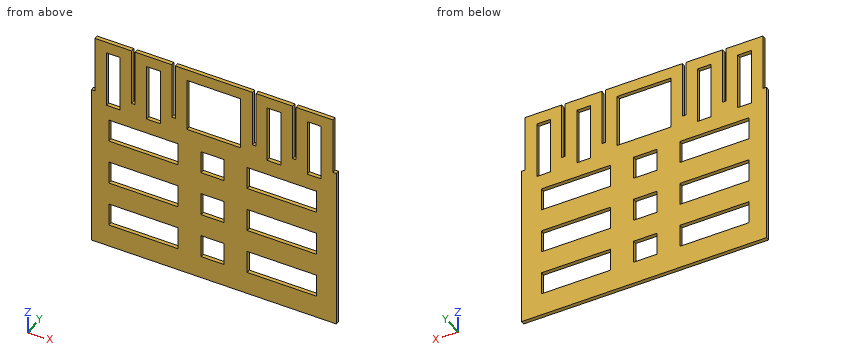
Autodesk Inventor part; units mm, degrees
ref_plane "YZ Plane" through (0, 0, 0) normal (1, 0, 0) x (0, 1, 0)
ref_plane "XZ Plane" through (0, 0, 0) normal (0, 1, 0) x (-1, 0, 0)
ref_plane "XY Plane" through (0, 0, 0) normal (0, 0, 1) x (1, 0, 0)
sketch "Sketch1" plane through (0, 0, 0) normal (0, 1, 0) x (-1, 0, 0)
  line L0 (0, 0) -> (318.5, 0)
  line L1 (318.5, 0) -> (318.5, -290)
  line L2 (318.5, -290) -> (0, -290)
  line L3 (0, -290) -> (0, 0)
  dimension "d0" = 318.5
  dimension "d1" = 290
extrude "Extrusion1" add sketch "Sketch1" along normal blind 5
sketch "Sketch2" plane through (0, 5, 0) normal (0, 1, 0) x (1, 0, 0)
  line L0 (0, 290) -> (-318.5, 290)
  line L1 (-318.5, 290) -> (-318.5, 75)
  line L2 (-318.5, 290) -> (-318.5, 0)
  line L3 (-318.5, 0) -> (0, 0)
  line L4 (-318.5, 75) -> (-314, 75)
  line L5 (-314, 75) -> (-314, 0)
  line L6 (-314, 0) -> (-318.5, 0)
  line L7 (-318.5, 0) -> (-318.5, 75)
  line L8 (-314, 75) -> (-266.25, 75)
  line L9 (-266.25, 75) -> (-261.75, 75)
  line L10 (-261.75, 75) -> (-261.75, 0)
  line L11 (-261.75, 0) -> (-266.25, 0)
  line L12 (-266.25, 0) -> (-266.25, 75)
  line L13 (-261.75, 75) -> (-214, 75)
  line L14 (-214, 75) -> (-209.5, 75)
  line L15 (-209.5, 75) -> (-209.5, 0)
  line L16 (-209.5, 0) -> (-214, 0)
  line L17 (-214, 0) -> (-214, 75)
  line L18 (-209.5, 75) -> (-162.03, 75)
  line L19 (-159.25, 290) -> (-159.25, 0)
  line L20 (0, 75) -> (-4.5, 75)
  line L21 (-4.5, 75) -> (-4.5, 0)
  line L22 (-4.5, 0) -> (0, 0)
  line L23 (0, 0) -> (0, 75)
  line L24 (-4.5, 75) -> (-52.25, 75)
  line L25 (-52.25, 75) -> (-56.75, 75)
  line L26 (-56.75, 75) -> (-56.75, 0)
  line L27 (-56.75, 0) -> (-52.25, 0)
  line L28 (-52.25, 0) -> (-52.25, 75)
  line L29 (-56.75, 75) -> (-104.5, 75)
  line L30 (-104.5, 75) -> (-109, 75)
  line L31 (-109, 75) -> (-109, 0)
  line L32 (-109, 0) -> (-104.5, 0)
  line L33 (-104.5, 0) -> (-104.5, 75)
  point P0 (-214, 0)
  point P1 (-266.25, 0)
  dimension "d4" = 215
  dimension "d5" = 4.5
  dimension "d6" = 47.75
  dimension "d7" = 4.5
  dimension "d8" = 47.75
  dimension "d9" = 4.5
  dimension "d10" = 47.47
extrude "Extrusion2" cut sketch "Sketch2" against normal blind 5 contours L31 L30 L33 L3 | L4 L5 L3 L2 | L3 L17 L14 L15 | L9 L10 L3 L12 | L26 L25 L28 L3 | L21 L20 L23 L3
sketch "Sketch3" plane through (0, 5, 0) normal (0, 1, 0) x (1, 0, 0)
  line L0 (-318.5, 290) -> (-318.5, 75)
  line L1 (-318.5, 290) -> (-296, 290)
  line L2 (-296, 290) -> (-296, 260)
  line L3 (-296, 260) -> (-318.5, 260)
  line L4 (-318.5, 260) -> (-318.5, 290)
  line L5 (-296, 260) -> (-266, 260)
  line L6 (-266, 260) -> (-266, 230)
  line L7 (-266, 230) -> (-296, 230)
  line L8 (-296, 230) -> (-296, 260)
  line L9 (-266, 200) -> (-266, 170)
  line L10 (-266, 170) -> (-296, 170)
  line L11 (-296, 170) -> (-296, 200)
  line L12 (-296, 200) -> (-266, 200)
  line L13 (-266, 140) -> (-266, 110)
  line L14 (-266, 110) -> (-296, 110)
  line L15 (-296, 110) -> (-296, 140)
  line L16 (-296, 140) -> (-266, 140)
  line L17 (-206, 260) -> (-206, 230)
  line L18 (-206, 230) -> (-236, 230)
  line L19 (-236, 230) -> (-236, 260)
  line L20 (-236, 260) -> (-206, 260)
  line L21 (-206, 200) -> (-206, 170)
  line L22 (-206, 170) -> (-236, 170)
  line L23 (-236, 170) -> (-236, 200)
  line L24 (-236, 200) -> (-206, 200)
  line L25 (-206, 140) -> (-206, 110)
  line L26 (-206, 110) -> (-236, 110)
  line L27 (-236, 110) -> (-236, 140)
  line L28 (-236, 140) -> (-206, 140)
  line L29 (-146, 260) -> (-146, 230)
  line L30 (-146, 230) -> (-176, 230)
  line L31 (-176, 230) -> (-176, 260)
  line L32 (-176, 260) -> (-146, 260)
  line L33 (-146, 200) -> (-146, 170)
  line L34 (-146, 170) -> (-176, 170)
  line L35 (-176, 170) -> (-176, 200)
  line L36 (-176, 200) -> (-146, 200)
  line L37 (-146, 140) -> (-146, 110)
  line L38 (-146, 110) -> (-176, 110)
  line L39 (-176, 110) -> (-176, 140)
  line L40 (-176, 140) -> (-146, 140)
  line L41 (-86, 260) -> (-86, 230)
  line L42 (-86, 230) -> (-116, 230)
  line L43 (-116, 230) -> (-116, 260)
  line L44 (-116, 260) -> (-86, 260)
  line L45 (-86, 200) -> (-86, 170)
  line L46 (-86, 170) -> (-116, 170)
  line L47 (-116, 170) -> (-116, 200)
  line L48 (-116, 200) -> (-86, 200)
  line L49 (-86, 140) -> (-86, 110)
  line L50 (-86, 110) -> (-116, 110)
  line L51 (-116, 110) -> (-116, 140)
  line L52 (-116, 140) -> (-86, 140)
  line L53 (-26, 260) -> (-26, 230)
  line L54 (-26, 230) -> (-56, 230)
  line L55 (-56, 230) -> (-56, 260)
  line L56 (-56, 260) -> (-26, 260)
  line L57 (-26, 200) -> (-26, 170)
  line L58 (-26, 170) -> (-56, 170)
  line L59 (-56, 170) -> (-56, 200)
  line L60 (-56, 200) -> (-26, 200)
  line L61 (-26, 140) -> (-26, 110)
  line L62 (-26, 110) -> (-56, 110)
  line L63 (-56, 110) -> (-56, 140)
  line L64 (-56, 140) -> (-26, 140)
  line L65 (-266, 200) -> (-236, 200)
  line L66 (-236, 200) -> (-236, 170)
  line L67 (-236, 170) -> (-266, 170)
  line L68 (-266, 170) -> (-266, 200)
  line L69 (-86, 200) -> (-56, 200)
  line L70 (-56, 200) -> (-56, 170)
  line L71 (-56, 170) -> (-86, 170)
  line L72 (-86, 170) -> (-86, 200)
  line L73 (-86, 260) -> (-56, 260)
  line L74 (-56, 260) -> (-56, 230)
  line L75 (-56, 230) -> (-86, 230)
  line L76 (-86, 230) -> (-86, 260)
  line L77 (-266, 260) -> (-236, 260)
  line L78 (-236, 260) -> (-236, 230)
  line L79 (-236, 230) -> (-266, 230)
  line L80 (-266, 230) -> (-266, 260)
  line L81 (-266, 140) -> (-236, 140)
  line L82 (-236, 140) -> (-236, 110)
  line L83 (-236, 110) -> (-266, 110)
  line L84 (-266, 110) -> (-266, 140)
  line L85 (-86, 140) -> (-56, 140)
  line L86 (-56, 140) -> (-56, 110)
  line L87 (-56, 110) -> (-86, 110)
  line L88 (-86, 110) -> (-86, 140)
  line L89 (-209.5, 0) -> (-109, 0)
  line L90 (-209.5, 0) -> (-194.5, 0)
  line L91 (-194.5, 0) -> (-194.5, 15)
  line L92 (-194.5, 15) -> (-209.5, 15)
  line L93 (-209.5, 15) -> (-209.5, 0)
  line L94 (-194.5, 15) -> (-124.5, 15)
  line L95 (-124.5, 15) -> (-124.5, 85)
  line L96 (-124.5, 85) -> (-194.5, 85)
  line L97 (-194.5, 85) -> (-194.5, 15)
  line L98 (-314, 0) -> (-314, 75)
  line L99 (-314, 0) -> (-299, 0)
  line L100 (-299, 0) -> (-299, 15)
  line L101 (-299, 15) -> (-314, 15)
  line L102 (-314, 15) -> (-314, 0)
  line L103 (-266.25, 75) -> (-266.25, 0)
  line L104 (-266.25, 75) -> (-281.25, 75)
  line L105 (-281.25, 75) -> (-281.25, 90)
  line L106 (-281.25, 90) -> (-266.25, 90)
  line L107 (-266.25, 90) -> (-266.25, 75)
  line L108 (-281.25, 90) -> (-299, 90)
  line L109 (-299, 90) -> (-299, 15)
  line L110 (-299, 15) -> (-281.25, 15)
  line L111 (-281.25, 15) -> (-281.25, 90)
  line L112 (-229, 15) -> (-229, 90)
  line L113 (-246.75, 90) -> (-246.75, 15)
  line L114 (-246.75, 15) -> (-229, 15)
  line L115 (-229, 90) -> (-246.75, 90)
  line L116 (-176.75, 15) -> (-176.75, 90)
  line L117 (-194.5, 90) -> (-194.5, 15)
  line L118 (-194.5, 15) -> (-176.75, 15)
  line L119 (-176.75, 90) -> (-194.5, 90)
  line L120 (-124.5, 15) -> (-124.5, 90)
  line L121 (-142.25, 90) -> (-142.25, 15)
  line L122 (-142.25, 15) -> (-124.5, 15)
  line L123 (-124.5, 90) -> (-142.25, 90)
  line L124 (-72.25, 15) -> (-72.25, 90)
  line L125 (-90, 90) -> (-90, 15)
  line L126 (-90, 15) -> (-72.25, 15)
  line L127 (-72.25, 90) -> (-90, 90)
  line L128 (-20, 15) -> (-20, 90)
  line L129 (-37.75, 90) -> (-37.75, 15)
  line L130 (-37.75, 15) -> (-20, 15)
  line L131 (-20, 90) -> (-37.75, 90)
  point P0 (-209.5, 75)
  dimension "d25" = 22.5
  dimension "d26" = 30
  dimension "d27" = 30
  dimension "d28" = 30
  dimension "d31" = 60
  dimension "d34" = 60
  dimension "d37" = 15
  dimension "d38" = 15
  dimension "d39" = 70
  dimension "d40" = 70
  dimension "d41" = 15
  dimension "d42" = 15
  dimension "d43" = 15
  dimension "d44" = 15
  dimension "d47" = 52.25
extrude "Extrusion3" cut sketch "Sketch3" against normal blind 5 contours L5 L6 L7 L8 | L77 L19 L79 L6 | L20 L17 L18 L19 | L65 L23 L67 L9 | L9 L10 L11 L12 | L24 L21 L22 L23 | L81 L27 L83 L13 | L13 L14 L15 L16 | L28 L25 L26 L27 | L29 L30 L31 L32 | L33 L34 L35 L36 | L37 L38 L39 L40 | L73 L55 L75 L41 | L41 L42 L43 L44 | L56 L53 L54 L55 | L69 L59 L71 L45 | L45 L46 L47 L48 | L60 L57 L58 L59 | L85 L63 L87 L49 | L49 L50 L51 L52 | L64 L61 L62 L63 | L97 L96 L116 L94 | L116 L96 L121 L94 | L121 L96 L95 L94 | L109 L108 L105 L111 L110 | L114 L113 L115 L112 | L126 L125 L127 L124 | L130 L129 L131 L128
properties part number "backrest" material "Foam Core Board"
Part model, mm, in its own coordinate system. Coordinates: 2 decimals unless noted, no trailing zeros. Write each loop counter-clockwise with the first axis right and the second up, starting at its lowest first coordinate (ties: lowest second). Pieces come first, ordered by that corner, then holes. Notation, with made-up numbers: (83.25, 64.5) - (125.25, 64.5) arc R15 ccw to (125.25, 68.5) - close; hole circle Ø5 at (89.25, 66). An arc over 180 degrees is marked (long way). Put each result on its own line as item: value.
1. Band-saw the part on A-A (x = -276.5). Write the cut outline in (y, z), then the cut area to 3 significant figures.
Final values:
outline: (0, -290) - (5, -290) - (5, -260) - (0, -260) - close; (0, -230) - (5, -230) - (5, -200) - (0, -200) - close; (0, -170) - (5, -170) - (5, -140) - (0, -140) - close; (0, -110) - (5, -110) - (5, 0) - (0, 0) - close
area: 1,000 mm²
2. Probe line 1 along Z through (x, y) = (-258.5, 3.65); line 2 along Z through (x, y) = (-293.5, 3.3); line 3 along X through (y, z) = (0.7, -190.5). List the from-to ranges inside material, lowest first. Write a range as [from, to].
Final values:
line 1: z = [-290, -260], [-230, -200], [-170, -140], [-110, 0]
line 2: z = [-290, -260], [-230, -200], [-170, -140], [-110, -90], [-15, 0]
line 3: x = [-318.5, -296], [-206, -176], [-146, -116], [-26, 0]
3. Band-saw the part on B-B (z = -78.5). Write the cut outline in (x, y).
Final values:
outline: (-318.5, 0) - (-299, 0) - (-299, 5) - (-318.5, 5) - close; (-281.25, 0) - (-246.75, 0) - (-246.75, 5) - (-281.25, 5) - close; (-229, 0) - (-194.5, 0) - (-194.5, 5) - (-229, 5) - close; (-124.5, 0) - (-90, 0) - (-90, 5) - (-124.5, 5) - close; (-72.25, 0) - (-37.75, 0) - (-37.75, 5) - (-72.25, 5) - close; (-20, 0) - (0, 0) - (0, 5) - (-20, 5) - close
4. Flat gauge pin, fed straight in: pin 1 Ø1.5 at (y, z) = (0.5, -49) entering from +X. Where does the tip first touch, or does it go through?
Final values:
pin 1: stops at x = -4.5
5. Band-saw the part on C-C (z = -128.5). Write the cut outline in (x, y).
Final values:
outline: (-318.5, 0) - (-296, 0) - (-296, 5) - (-318.5, 5) - close; (-206, 0) - (-176, 0) - (-176, 5) - (-206, 5) - close; (-146, 0) - (-116, 0) - (-116, 5) - (-146, 5) - close; (-26, 0) - (0, 0) - (0, 5) - (-26, 5) - close
6. Band-saw the part on D-D (y = 3.9). Give the number of separate pieces and of enclosed holes in the cut face, then the cut area to 3 significant figures.
Final values:
separate pieces: 1
enclosed holes: 14
area: 61,200 mm²
